Can you work these out from the model? Positions are in its coordinate system, mm. Round coordinates to 2 decimals unless told otherwise and drop trailing zeros. Loops run counter-clockwise (first coordinate to the right, second up) from the corner with the lowest first, then second, coordinate; pieces in that order, holes last.
(1) If I drill on line 1 along Y through (x, z) = (-48, 3.05); line 2 along Y through (x, z) = (1.5, 2.5); line 3 along Y through (x, z) = (0, 3.4), over which ranges is the centre line in solid material (lowest first)?
(2) I want a section at D-D on y = -12. Write out the boundary of the cut face in (x, z).
(3) I want a section at C-C on z = 2.15. Write out the boundary of the cut face in (x, y), plus the area to 3 significant figures.
(4) I want a section at B-B on x = -12. Write out the boundary of the cut face in (y, z), plus the area to 3 significant figures.
(5) I want a section at A-A on y = 28. Write out the boundary of the cut face in (x, z).
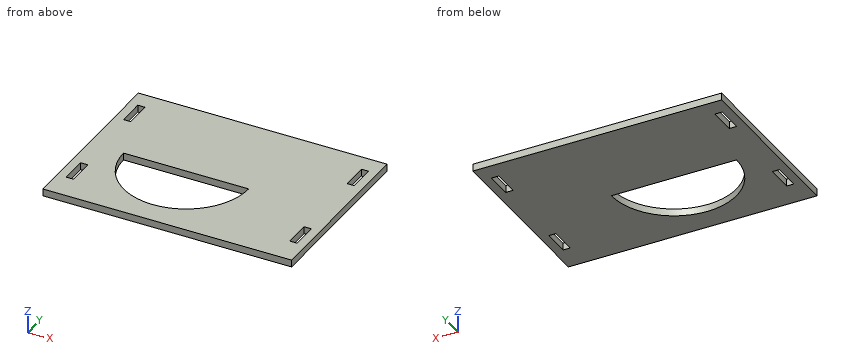
from build123d import *

# Parameters (mm, degrees)
SKETCH1_W           = 4
SKETCH1_H           = 15
BOSS_EXTRUDE1_DEPTH = 4


with BuildPart() as part:
    # Sketch1 → Boss-Extrude1 (new body)
    with BuildSketch(Plane.XY):
        Polygon((-54.5, -52.5), (64.5, -52.5), (84.5, -52.5), (84.5, 47.5), (64.5, 47.5), (-54.5, 47.5), align=None)
        with BuildLine():
            Line((-35, -4.678634488), (35, -4.678634488))
            ThreePointArc((35, -4.678634488), (0, -39.678634488), (-35, -4.678634488))
        make_face(mode=Mode.SUBTRACT)
        with Locations((-47.5, -30)):
            Rectangle(SKETCH1_W, SKETCH1_H, mode=Mode.SUBTRACT)
        with Locations((-47.5, 30)):
            Rectangle(SKETCH1_W, SKETCH1_H, mode=Mode.SUBTRACT)
        with Locations((77.5, 30)):
            Rectangle(SKETCH1_W, SKETCH1_H, mode=Mode.SUBTRACT)
        with Locations((77.5, -30)):
            Rectangle(SKETCH1_W, SKETCH1_H, mode=Mode.SUBTRACT)
    extrude(amount=BOSS_EXTRUDE1_DEPTH)


solid = part.part
Filled sheet:
1. line 1: y = -52.5 to -37.5, -22.5 to 22.5, 37.5 to 47.5
1. line 2: y = -52.5 to -39.65, -4.68 to 47.5
1. line 3: y = -52.5 to -39.68, -4.68 to 47.5
2. outline: (-54.5, 0) - (-34.23, 0) - (-34.23, 4) - (-54.5, 4) - close; (34.23, 0) - (84.5, 0) - (84.5, 4) - (34.23, 4) - close
3. outline: (-54.5, -52.5) - (84.5, -52.5) - (84.5, 47.5) - (-54.5, 47.5) - close; hole (-49.5, -37.5) - (-45.5, -37.5) - (-45.5, -22.5) - (-49.5, -22.5) - close; hole (-49.5, 22.5) - (-45.5, 22.5) - (-45.5, 37.5) - (-49.5, 37.5) - close; hole (-35, -4.68) arc R35 ccw to (35, -4.68) - close; hole (75.5, -37.5) - (79.5, -37.5) - (79.5, -22.5) - (75.5, -22.5) - close; hole (75.5, 22.5) - (79.5, 22.5) - (79.5, 37.5) - (75.5, 37.5) - close
3. area: 11,700 mm2
4. outline: (-52.5, 0) - (-37.56, 0) - (-37.56, 4) - (-52.5, 4) - close; (-4.68, 0) - (47.5, 0) - (47.5, 4) - (-4.68, 4) - close
4. area: 268 mm2
5. outline: (-54.5, 0) - (-49.5, 0) - (-49.5, 4) - (-54.5, 4) - close; (-45.5, 0) - (75.5, 0) - (75.5, 4) - (-45.5, 4) - close; (79.5, 0) - (84.5, 0) - (84.5, 4) - (79.5, 4) - close
